Build history of the part. All positions in model axes, mm. Face numbers are marked on the shaded views. A direction names the side the tool comes from. Give positions to 0.01 mm unless a question says otherwise; leave off trailing zeros. Write each loop counter-clockwise with the first axis right and the second up, starting at its lowest first coordinate (ties: lowest second). Pieces come first, ordered by that corner, then holes. Notation, with made-up numbers: (8, 54.5) -> (46, 54.5) arc R29 ccw to (46, 93.5) -> close; hole circle Ø2 at (74.25, -27). An arc over 180 degrees is marked (long way). Put each result on its own line as item: value.
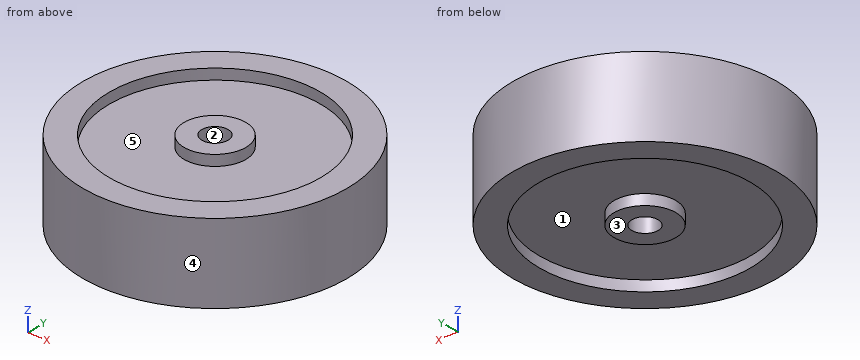
Autodesk Inventor part; units mm, degrees
ref_plane "YZ Plane" through (0, 0, 0) normal (1, 0, 0) x (0, 1, 0)
ref_plane "XZ Plane" through (0, 0, 0) normal (0, 1, 0) x (-1, 0, 0)
ref_plane "XY Plane" through (0, 0, 0) normal (0, 0, 1) x (1, 0, 0)
sketch "Sketch3" plane through (0, 0, 0) normal (0, 0, 1) x (1, 0, 0)
  circle A0 centre (0, 0) radius 63.5
  dimension "d1" = 127
extrude "Extrusion1" add sketch "Sketch3" along normal blind 38.1
sketch "Sketch4" plane through (0, 0, 38.1) normal (0, 0, 1) x (1, 0, 0)
  circle A0 centre (0, 0) radius 6.35
  dimension "d4" = 12.7
hole "Hole1" at (0, 0, 38.1) direction (0, 0, -1) diameter 12.7 end through all
sketch "Sketch5" plane through (0, 0, 38.1) normal (0, 0, 1) x (1, 0, 0)
  circle A0 centre (0, 0) radius 50.8
  circle A1 centre (0, 0) radius 14.861
  dimension "d12" = 101.6
  dimension "d13" = 29.722
emboss "Emboss1" sketch "Sketch5" operation cut depth 5.08 direction (0, 0, -1)
sketch "Sketch6" plane through (0, 0, 0) normal (0, 0, -1) x (-1, 0, 0)
  circle A0 centre (0, 0) radius 50.8
  circle A1 centre (0, 0) radius 14.861
  dimension "d16" = 101.6
  dimension "d17" = 29.722
emboss "Emboss2" sketch "Sketch6" operation cut depth 5.08 direction (0, 0, 1)
properties part number "SubWheelWithHole"
1) Slice it at A-A (x = 0). Write the cut outline in (y, z), plus the area to 3 significant figures.
Filled sheet:
outline: (-63.5, 0) -> (-50.8, 0) -> (-50.8, 5.08) -> (-14.86, 5.08) -> (-14.86, 0) -> (-6.35, 0) -> (-6.35, 38.1) -> (-14.86, 38.1) -> (-14.86, 33.02) -> (-50.8, 33.02) -> (-50.8, 38.1) -> (-63.5, 38.1) -> close; (6.35, 0) -> (14.86, 0) -> (14.86, 5.08) -> (50.8, 5.08) -> (50.8, 0) -> (63.5, 0) -> (63.5, 38.1) -> (50.8, 38.1) -> (50.8, 33.02) -> (14.86, 33.02) -> (14.86, 38.1) -> (6.35, 38.1) -> close
area: 3,620 mm2
2) Tool access for the marked faces 1 and 2: list every direction of +Z, -Z, +X, -X, +Y, -Y with a clear straight run to the whole face (end or side of a thin tool).
Filled sheet:
face 1: -Z
face 2: +Z, -Z
3) Wall check: L1, parallel to Y at x = 0, z = 35; L2, parallel to X at y = 13, z = 35; L3, parallel to Z at x = -20.5, y = -36. Give the ranges that are in metal, low to high.
Filled sheet:
L1: -63.5 to -50.8, -14.86 to -6.35, 6.35 to 14.86, 50.8 to 63.5
L2: -62.16 to -49.11, -7.2 to 7.2, 49.11 to 62.16
L3: 5.08 to 33.02
4) Slice it at D-D (z = 23). Write the cut outline in (x, y).
Filled sheet:
outline: circle Ø127 at (0, 0); hole circle Ø12.7 at (0, 0)
5) Slice it at C-C (y = -17.5). Write the cut outline in (x, z), plus the area to 3 significant figures.
Filled sheet:
outline: (-61.04, 0) -> (-47.69, 0) -> (-47.69, 5.08) -> (47.69, 5.08) -> (47.69, 0) -> (61.04, 0) -> (61.04, 38.1) -> (47.69, 38.1) -> (47.69, 33.02) -> (-47.69, 33.02) -> (-47.69, 38.1) -> (-61.04, 38.1) -> close
area: 3,680 mm2
6) Pin check, flat tips, straight feed: pin 1 (16.5 mm diameter, centred on x = 0, y = 0, fed in from +Z); pin 2 (1.5 mm diameter, centred on y = 48.5, z = 33.5, fed in from -X); pin 3 (1 mm diameter, centred on y = 1.5, z = 19, fed in from -X); pin 4 (6 mm diameter, centred on x = -15, z = 17.5, fed in from -Y). Stop position of each tip, or through.
Filled sheet:
pin 1: z = 38.1
pin 2: x = -41.86
pin 3: x = -63.49
pin 4: y = -62.36
7) Pull direction Y, two halves, no side cores. Call the marked faces 3, 4 and 5: released by +Y, released by -Y, zero draft, split by the parting line, or undercut.
Filled sheet:
face 3: zero draft
face 4: split by the parting line
face 5: undercut
